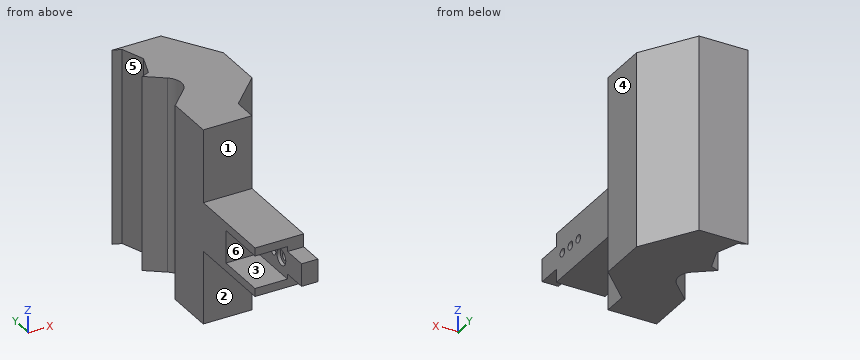
Autodesk Inventor part; units mm, degrees
ref_plane "Work Plane1" through (0, 0, -15) normal (0, 0, 1) x (1, 0, 0)
ref_plane "YZ Plane" through (0, 0, 0) normal (1, 0, 0) x (0, 1, 0)
ref_plane "XZ Plane" through (0, 0, 0) normal (0, 1, 0) x (-1, 0, 0)
sketch "Sketch1" plane through (0, 0, 0) normal (0, 0, 1) x (1, 0, 0)
  line L0 (0, 0) -> (25, 0)
  line L1 (25, 0) -> (25, 40)
  line L2 (25, 40) -> (0, 40)
  line L3 (0, 40) -> (0, 0)
  dimension "d1" = 25
  dimension "d2" = 40
  dimension "d3" = 25
extrude "Extrusion1" add sketch "Sketch1" against normal blind 30
sketch "Sketch2" plane through (25, 0, 0) normal (1, 0, 0) x (0, 0, -1)
  line L0 (0, 0) -> (30, 0)
  circle A0 centre (15, 6.56) radius 2.46
extrude "Extrusion2" cut sketch "Sketch2" against normal blind 30
sketch "Sketch3" plane through (0, 0, 0) normal (-1, 0, 0) x (0, 0, 1)
  line L0 (0, 0) -> (-30, 0)
  line L1 (-25.05, 0) -> (-4.95, 0)
  line L2 (-4.95, 0) -> (-4.95, 33.12)
  line L3 (-4.95, 33.12) -> (-25.05, 33.12)
  line L4 (-25.05, 33.12) -> (-25.05, 0)
  dimension "d11" = 20.1
extrude "Extrusion3" cut sketch "Sketch3" against normal blind 20
sketch "Sketch4" plane through (0, 0, 0) normal (0, -1, 0) x (1, 0, 0)
  line L0 (20, -4.95) -> (20, -25.05)
  line L1 (20, -15) -> (25, -15)
  line L2 (25, 0) -> (25, -30)
  line L3 (20, -8.025) -> (25, -8.025)
  line L4 (25, -8.025) -> (25, -21.975)
  line L5 (25, -21.975) -> (20, -21.975)
  line L6 (20, -21.975) -> (20, -8.025)
  line L7 (20, -8.025) -> (25, -21.975) construction
  line L8 (25, -8.025) -> (20, -21.975) construction
  line L9 (25, -12.54) -> (25, -17.46)
  point P0 (0, 0)
  point P1 (22.5, -15)
  dimension "d14" = 13.95
extrude "Extrusion4" add sketch "Sketch4" along normal blind 15
sketch "Sketch5" plane through (20, 0, 0) normal (-1, 0, 0) x (0, 0, 1)
  circle A0 centre (-15, 6.56) radius 2.46
  circle A1 centre (-15, 6.56) radius 4.7025
  circle A2 centre (-15, 6.56) radius 2.46
  circle A3 centre (-15, 6.56) radius 2.46
  point P0 (0, 0)
  dimension "d17" = 9.405
extrude "Extrusion5" cut sketch "Sketch5" against normal blind 2.1
sketch "Sketch6" plane through (25, 0, 0) normal (1, 0, 0) x (0, 0, -1)
  circle A0 centre (15, 6.56) radius 4.7025
  line L0 (15, 6.56) -> (15, 23.56)
  circle A1 centre (15, 23.56) radius 2.46
  point P0 (0, 0)
  dimension "d20" = 17
  dimension "d21" = 4.92
extrude "Extrusion6" cut sketch "Sketch6" against normal blind 10 contours A1
sketch "Sketch7" plane through (20, 0, 0) normal (-1, 0, 0) x (0, 0, 1)
  circle A0 centre (-15, 23.56) radius 2.46
  circle A1 centre (-15, 23.56) radius 4.7025
  point P0 (0, 0)
  dimension "d24" = 9.405
extrude "Extrusion7" cut sketch "Sketch7" against normal blind 2.1
sketch "Sketch9" plane through (25, 0, 0) normal (1, 0, 0) x (0, 0, -1)
  circle A0 centre (15, 6.56) radius 2.46
  circle A1 centre (15, 6.56) radius 2.46
  circle A2 centre (15, 23.56) radius 2.46
  circle A3 centre (15, 23.56) radius 2.46
  line L0 (30, 40) -> (30, 0)
  line L1 (30, 0) -> (30, 40)
  line L2 (30, 40) -> (0, 40)
  line L3 (0, 40) -> (0, 0)
  line L4 (0, 0) -> (8.025, 0)
  line L5 (21.975, 0) -> (21.975, -15)
  line L6 (21.975, -15) -> (8.025, -15)
  line L7 (8.025, -15) -> (8.025, 0)
  line L8 (0, 0) -> (8.025, 0)
  line L9 (21.975, 0) -> (30, 0)
extrude "Extrusion8" add sketch "Sketch9" along normal blind 5
sketch "Sketch10" plane through (0, 40, 0) normal (0, 1, 0) x (1, 0, 0)
  line L0 (0, 30) -> (30, 30)
  line L1 (30, 0) -> (0, 0)
  line L2 (0, 30) -> (30, 30)
  line L3 (30, 30) -> (30, 0)
  line L4 (30, 0) -> (0, 0)
  line L5 (0, 0) -> (0, 30)
extrude "Extrusion9" add sketch "Sketch10" along normal blind 30
sketch "Sketch12" plane through (30, 0, 0) normal (1, 0, 0) x (0, 0, -1)
  circle A0 centre (15, 6.56) radius 2.46
  line L0 (15, 6.56) -> (15, 15.06)
  circle A1 centre (15, 15.06) radius 2.525
  point P0 (0, 0)
  dimension "d31" = 8.5
  dimension "d33" = 5.05
extrude "Extrusion10" cut sketch "Sketch12" against normal blind 30 contours A1
sketch "Sketch15" plane through (0, 0, -25.05) normal (-1, 0, 0) x (0, 0, 1)
  line L0 (0, 33.12) -> (20.1, 33.12)
  line L1 (20.1, 33.12) -> (20.1, 0)
  line L2 (0, 33.12) -> (20.1, 33.12)
  line L3 (20.1, 33.12) -> (20.1, 31.1)
  line L4 (20.1, 31.1) -> (0, 31.1)
  line L5 (0, 31.1) -> (0, 33.12)
  point P0 (25.05, 0)
  dimension "d57" = 2.02
extrude "Extrusion13" add sketch "Sketch15" against normal blind 20
sketch "Sketch17" plane through (0, 0, 0) normal (0, 0, 1) x (1, 0, 0)
  line L0 (0, 70) -> (30, 70)
  line L1 (30, 70) -> (50.0622, 90.0622)
  line L2 (30, 70) -> (80, 70) construction
  line L3 (11.9522, 97.2454) -> (0, 85.2932)
  line L4 (0, 70) -> (0, 85.2932)
  line L5 (0, 70) -> (0, 0)
  line L6 (0, 70) -> (30, 70)
  line L7 (10.923, 112.2849) -> (0, 120.567)
  line L8 (50.0622, 105.3553) -> (50.0622, 120.567)
  line L9 (50.0622, 105.3553) -> (50.0622, 90.0622)
  arc A0 (11.9522, 97.2454) -> (10.923, 112.2849) centre (4.8811, 104.3165) ccw
  line L10 (0, 152.567) -> (30, 152.567)
  line L11 (30, 152.567) -> (50.0622, 120.567)
  line L12 (5, 150.567) -> (0, 152.567)
  line L13 (5, 122.567) -> (0, 120.567)
  line L14 (5, 122.567) -> (10, 136.567)
  line L15 (10, 136.567) -> (5, 150.567)
  dimension "d61" = 45
  dimension "d62" = 32.0271
  dimension "d72" = 10
extrude "Extrusion14" add sketch "Sketch17" against normal blind 30
sketch "Sketch22" plane through (0, 0, 0) normal (0, 0, 1) x (1, 0, 0)
  line L0 (30, 0) -> (30, 70)
  line L1 (50.0622, 90.0622) -> (30, 70)
  line L2 (30, 70) -> (50.0622, 90.0622)
  line L3 (50.0622, 120.567) -> (50.0622, 90.0622)
  line L4 (50.0622, 90.0622) -> (50.0622, 120.567)
  line L5 (30, 152.567) -> (50.0622, 120.567)
  line L6 (50.0622, 120.567) -> (30, 152.567)
  line L7 (0, 152.567) -> (30, 152.567)
  line L8 (30, 152.567) -> (0, 152.567)
  line L9 (5, 150.567) -> (0, 152.567)
  line L10 (0, 152.567) -> (5, 150.567)
  line L11 (5, 150.567) -> (10, 136.567)
  line L12 (5, 150.567) -> (10, 136.567)
  line L13 (10, 136.567) -> (5, 122.567)
  line L14 (10, 136.567) -> (5, 122.567)
  line L15 (5, 122.567) -> (0, 120.567)
  line L16 (5, 122.567) -> (0, 120.567)
  line L17 (0, 120.567) -> (10.923, 112.2849)
  line L18 (0, 120.567) -> (10.923, 112.2849)
  line L19 (0, 85.2932) -> (11.9522, 97.2454)
  line L20 (11.9522, 97.2454) -> (0, 85.2932)
  line L21 (0, 85.2932) -> (0, 55.2932)
  line L22 (0, 0) -> (0, 85.2932)
  line L23 (0, 55.2932) -> (30, 55.2932)
  line L24 (30, 55.2932) -> (30, 70)
  arc A0 (11.9522, 97.2454) -> (10.923, 112.2849) centre (4.8811, 104.3165) ccw
  dimension "d92" = 30
extrude "Extrusion15" add sketch "Sketch22" along normal blind 45
ref_plane "Work Plane1" through (0, 0, -15) normal (0, 0, 1) x (1, 0, 0)
mirror "Mirror1" about plane through (0, 0, -15) normal (0, 0, 1) of "Extrusion15"
properties part number "rec_c_28mm_x_120mm"
Work out the finished part from the listing and answer in its coordinate system (mm). Face numbers are marked on the shaded views. A direction names the side the tool comes from. Give positions to 0.01 mm unless a question says otherwise; leave off trailing zeros. Loops run counter-clockwise (first coordinate to the right, second up) from the corner with the lowest first, then second, coordinate; pieces in that order, holes last. Notation, with made-up numbers: (82, 39.5) -> (112, 39.5) arc R18 ccw to (112, 60.5) -> close; hole circle Ø8 at (-10, -19.5). An arc over 180 degrees is marked (long way). Use CSV: the item, a comma, the result in double quotes.
1. The part is cut by section A-A (y = 23.56). Write down the section's boundary in (x, z), then the cut area to 3 significant figures.
Found:
outline,"(0, -30) -> (30, -30) -> (30, -17.46) -> (22.1, -17.46) -> (22.1, -19.7) -> (20, -19.7) -> (20, -25.05) -> (0, -25.05) -> close; (0, -4.95) -> (20, -4.95) -> (20, -10.3) -> (22.1, -10.3) -> (22.1, -12.54) -> (30, -12.54) -> (30, 0) -> (0, 0) -> close"
area,"439 mm^2"
2. The part is cut by section D-D (x = 38). Write down the section's boundary in (y, z), then the cut area to 3 significant figures.
Found:
outline,"(78, -75) -> (139.81, -75) -> (139.81, 45) -> (78, 45) -> close"
area,"7,420 mm^2"
3. Straight lines are drawn through the part: line 1 (Y direction, x = 24, z = -15) (3 decimals); line 2 (Z direction, x = 24.5, y = 6.56); line 3 (X direction, y = 39.5, z = -8.5). For each, find the intervals that lie inside material, in ascending order.
Found:
line 1,"-15 to 4.1, 9.02 to 12.535, 17.585 to 21.1, 26.02 to 152.567"
line 2,"-30 to -17.46, -12.54 to 0"
line 3,"0 to 30"
4. Flat-ended cylindrical pins translate along their axes: pin 1 Ø11 at (y, z) = (6.56, -15) entering from -X; pin 2 Ø6 at (x, y) = (9.5, 16) entering from -Z; pin 3 Ø3 at (x, y) = (24.5, -7) entering from +Z (3 decimals). Find the tip coordinate at first contact, or state that the pin passes through.
Found:
pin 1,"x = 20"
pin 2,"z = -30"
pin 3,"z = -8.025"
5. The part is cut by section B-B (z = 6.5). Write down the section's boundary in (x, y), then the cut area to 3 significant figures.
Found:
outline,"(0, 55.29) -> (30, 55.29) -> (30, 70) -> (50.06, 90.06) -> (50.06, 120.57) -> (30, 152.57) -> (0, 152.57) -> (5, 150.57) -> (10, 136.57) -> (5, 122.57) -> (0, 120.57) -> (10.92, 112.28) arc R10 cw to (11.95, 97.25) -> (0, 85.29) -> close"
area,"3,510 mm^2"
6. A tool of negligible diameter and unlimited length cuts with its end or side. For the marked faces 1, 2 and 3, from which of +Z, -Z, +X, -X, +Y, -Y can it reach the whole face along a straight path? Write none if from no direction.
Found:
face 1,"+Z, +X, -X, -Y"
face 2,"-Z, +X, -X, -Y"
face 3,"-X, -Y"
7. The mould has two halves that part along Y. Classify the marked faces 4, 5 and 6: +Y half, -Y half, draft (parallel to the pull), parting line (faces both ways), or undercut.
Found:
face 4,"draft"
face 5,"undercut"
face 6,"-Y half"
8. The part is cut by section C-C (z = -15). State how many separate pieces and enclosed holes the cut face has, then the cut area to 3 significant figures.
Found:
separate pieces,"4"
enclosed holes,"0"
area,"4,530 mm^2"
